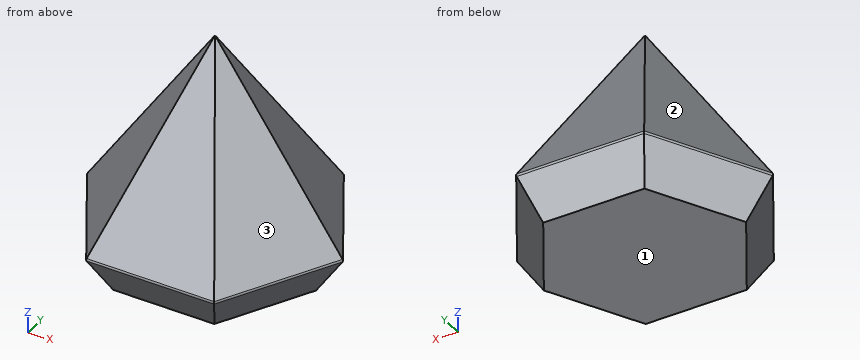
```python
from build123d import *

# Parameters (mm, degrees)
F1_DEPTH = 15
F1_TAPER = -30
F2_DEPTH = 15
F2_TAPER = -30
F3_DEPTH = 1
F3_TAPER = -35
F5_DEPTH = 70
F5_TAPER = 30
F9_R     = 1


# Not quite as in the source:
# - an extrude whose draft closes it to a point is written as a loft to that point


with BuildPart() as f1:
    # F0 (on Top) → F1 (new body)
    with BuildSketch(Plane.XY):
        Polygon((-18.4989116336, 32.043568284), (-36.9999999787, 0.0012567249), (-18.501088345, -32.0423115591), (18.4989116336, -32.043568284), (36.9999999787, -0.0012567249), (18.501088345, 32.0423115591), align=None)
        Polygon((17.57727357, 30.442342936), (35.1524791183, -0.0011939729), (17.5752055483, -30.4435369089), (-17.57727357, -30.442342936), (-35.1524791183, 0.0011939729), (-17.5752055483, 30.4435369089), align=None, mode=Mode.SUBTRACT)
    extrude(amount=F1_DEPTH, taper=F1_TAPER)

    # F0 (on Top) → F2 (cut)
    with BuildSketch(Plane.XY):
        Polygon((17.5752055483, -30.4435369089), (35.1524791183, -0.0011939729), (17.57727357, 30.442342936), (-17.5752055483, 30.4435369089), (-35.1524791183, 0.0011939729), (-17.57727357, -30.442342936), align=None)
    extrude(amount=F2_DEPTH, taper=F2_TAPER, mode=Mode.SUBTRACT)

    # F0 (on Top) → F3 (join)
    with BuildSketch(Plane.XY):
        Polygon((17.5752055483, -30.4435369089), (35.1524791183, -0.0011939729), (17.57727357, 30.442342936), (-17.5752055483, 30.4435369089), (-35.1524791183, 0.0011939729), (-17.57727357, -30.442342936), align=None)
    extrude(amount=F3_DEPTH, taper=F3_TAPER)


with BuildPart() as f5:
    # F4 (on face) → F5 (new body)
    with BuildSketch(Plane.XY.offset(15)):
        Polygon((23.4986174805, -40.7039921445), (46.9999999729, -0.0015963803), (23.5013824923, 40.7023957642), (-23.4986174805, 40.7039921445), (-46.9999999729, 0.0015963803), (-23.5013824923, -40.7023957642), align=None)
    extrude(amount=F5_DEPTH, taper=F5_TAPER)

    # F6 (on face) → F7 section 0
    with BuildSketch(Plane(origin=(0, 0, 15), x_dir=(1, 0, 0), z_dir=(0, 0, -1)), mode=Mode.PRIVATE) as f7_s0:
        Polygon((45.3999999738, 0.0015420354), (22.698664545, 39.3183243269), (-22.7013354288, 39.3167822914), (-45.3999999738, -0.0015420354), (-22.698664545, -39.3183243269), (22.7013354288, -39.3167822914), align=None)
    loft([f7_s0.sketch, Vertex(0, 0, 83.1)], ruled=True, mode=Mode.SUBTRACT)


with BuildPart() as f1_1:
    add(f1.part)

    # F8: union F5
    add(f5.part)

    # F9
    f9_edges = [f1_1.edges().sort_by_distance(p)[0] for p in [
        (-0.001383, -40.703194, 15),
        (35.249309, -20.352794, 15),
        (35.250691, 20.3504, 15),
        (0.001383, 40.703194, 15),
        (-35.249309, 20.352794, 15),
        (-35.250691, -20.3504, 15),
    ]]
    fillet(f9_edges, radius=F9_R)


solid = f1_1.part
```
CAD build for the part. Positions are in the model's coordinates, mm. Face numbers are marked on the shaded views. Give positions to 0.01 mm unless a question says otherwise; leave off trailing zeros. Write each loop counter-clockwise with the first axis right and the second up, starting at its lowest first coordinate (ties: lowest second). Pieces come first, ordered by that corner, then holes. Notation, with made-up numbers: M 79,61 L 108,61 A22 cw 108,79 Z; hole C 37,-8 d7. An arc over 180 degrees is marked long. Return JSON: item names as keys, results as strings. Group by question number.
(1) Band-saw the part on A-A (z = 79.5). Give the cut face in (x, y).
(2) Mould opens along X. For the marked faces 1, 2 and 3 say: pulls with the +X half, pulls with the -X half, needs draft (parallel to the pull), parting line crosses it, or undercut.
(3) Flat gauge pins, fed straight in: pin 1 Ø1.5 at (y, z) = (8, 62) entering from +X; pin 2 Ø3 at (x, y) = (-31.5, 15) entering from -Z; pin 3 Ø6 at (y, z) = (22.5, 31.5) entering from +X. Where does each tip first touch, or does it go through?
(4) Drill centre lines: L1, parallel to X at y = 15, z = 30; L2, parallel to Y at x = -37.5, z = 18.5; L3, parallel to Z at x = -15.5, y = -1.5. Where is each one in solid material? Low to high. Write a range as [from, to].
(5) Band-saw the part on B-B (z = 40). Give the cut face in (x, y), and give its area (3 significant figures).
Entries:
{
 "1": {"outline": "M -4,0 L -2,-3.46 L 2,-3.46 L 4,0 L 2,3.46 L -2,3.46 Z; hole M -2.4,0 L -1.2,-2.08 L 1.2,-2.08 L 2.4,0 L 1.2,2.08 L -1.2,2.08 Z"},
 "2": {"face 1": "needs draft", "face 2": "pulls with the -X half", "face 3": "pulls with the +X half"},
 "3": {"pin 1": "stops at x = 11.71", "pin 2": "stops at z = 2.14", "pin 3": "stops at x = 25.66"},
 "4": {"L1": "x = [-28.34, -26.74], [26.74, 28.34]", "L2": "y = [-12.41, -9.64], [9.64, 12.41]", "L3": "z = [0, 1], [58.55, 60.95]"},
 "5": {"outline": "M -30.33,0 L -15.17,-26.27 L 15.17,-26.27 L 30.33,0 L 15.17,26.27 L -15.17,26.27 Z; hole M -28.73,0 L -14.37,-24.88 L 14.37,-24.88 L 28.73,0 L 14.37,24.88 L -14.37,24.88 Z", "area": "246 mm^2"}
}
